Build history of the part. All positions in model axes, mm. Face numbers are marked on the shaded views. A direction names the side the tool comes from. Round coordinates to 2 decimals unless told otherwise and drop trailing zeros. Write each loop counter-clockwise with the first axis right and the second up, starting at its lowest first coordinate (ties: lowest second). Pieces come first, ordered by that corner, then holes.
1) Flat gauge pins, fed straight in: pin 1 (5 mm diameter, centred on x = 8.5, z = -17.5, fed in from -Y); pin 2 (0.5 mm diameter, centred on x = -14.5, z = 0.5, fed in from +Y); pin 3 (11 mm diameter, centred on x = 6, y = -8, fed in from -Z). Where does each tip first touch, or does it go through?
2) Saw through at B-B (y = -2). Write the cut outline in (x, z).
3) Saw through at C-C (z = -22). Write the cut outline in (x, y), plus the area to 3 significant figures.
4) Wall check: probe 1 along Y at (x, z) = (13, -6); probe 2 along Z at (x, y) = (-1, -4). Give the ranges that are in metal, low to high.
5) Saw through at A-A (x = 16). Write the cut outline in (y, z), plus the area to 3 significant figures.
6) Which spindle directions (+Z, -Z, +X, -X, +Y, -Y) get a long thin tool onto all of the face, cutting with end or side? Do the marked faces 1 and 2. Say none if no direction does.
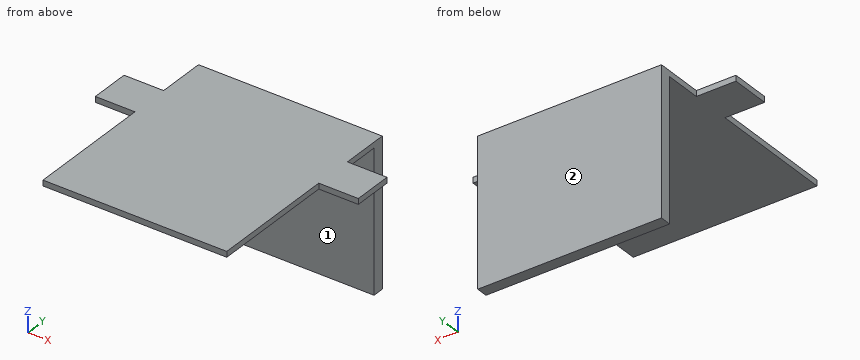
Autodesk Inventor part; units mm, degrees
ref_plane "YZ Plane" through (0, 0, 0) normal (1, 0, 0) x (0, 1, 0)
ref_plane "XZ Plane" through (0, 0, 0) normal (0, 1, 0) x (-1, 0, 0)
ref_plane "XY Plane" through (0, 0, 0) normal (0, 0, 1) x (1, 0, 0)
sketch "Sketch1" plane through (0, 0, 0) normal (0, 0, 1) x (1, 0, 0)
  line L0 (-10.2966, 10.8783) -> (22.1834, 10.8783)
  line L1 (22.1834, 10.8783) -> (22.1834, -25.1217)
  line L2 (22.1834, -25.1217) -> (-10.2966, -25.1217)
  line L3 (-10.2966, -25.1217) -> (-10.2966, 10.8783)
  line L4 (-10.2966, -25.1217) -> (-10.2966, -2.6417)
  line L5 (-10.2966, -2.6417) -> (-17.2966, -2.6417)
  line L6 (-17.2966, -2.6417) -> (-17.2966, 4.3583)
  line L7 (-17.2966, 4.3583) -> (-10.2966, 4.3583)
  line L8 (22.1834, 4.3583) -> (29.1834, 4.3583)
  line L9 (29.1834, 4.3583) -> (29.1834, -2.6417)
  line L10 (29.1834, -2.6417) -> (22.1834, -2.6417)
  line L11 (-10.2966, 10.8783) -> (-10.2966, 12.8783)
  line L12 (-10.2966, 12.8783) -> (22.1834, 12.8783)
  line L13 (22.1834, 12.8783) -> (22.1834, 10.8783)
  point P0 (0, 0)
  dimension "d0" = 32.48
  dimension "d1" = 36
  dimension "d2" = 22.48
  dimension "d3" = 7
  dimension "d4" = 90
  dimension "d5" = 7
  dimension "d6" = 7
  dimension "d7" = 2
extrude "Extrusion1" add sketch "Sketch1" along normal blind 1
extrude "Extrusion2" add sketch "Sketch1" against normal blind 25 contours L11 L12 L13 L0
properties part number "shell 6.0 cover"
Evaluation:
1. pin 1: stops at y = 10.88
1. pin 2: stops at y = 4.36
1. pin 3: stops at z = 0
2. outline: (-17.3, 0) - (29.18, 0) - (29.18, 1) - (-17.3, 1) - close
3. outline: (-10.3, 10.88) - (22.18, 10.88) - (22.18, 12.88) - (-10.3, 12.88) - close
3. area: 65.0 mm2
4. probe 1: y = 10.88 to 12.88
4. probe 2: z = 0 to 1
5. outline: (-25.12, 0) - (10.88, 0) - (10.88, -25) - (12.88, -25) - (12.88, 1) - (-25.12, 1) - close
5. area: 88.0 mm2
6. face 1: -Z, +X, -X, -Y
6. face 2: +Z, -Z, +X, -X, +Y
